Source: three-view drawing plus pictorial views. Frame: mm from the lowest corner of the part. A direction names the side the tool comes from. Give positions to 0.01 mm unless a question says otherwise; leave off trailing zeros. Write each loop counter-clockwise with the first axis right and the second up, starting at its lowest first coordinate (ties: lowest second). Pieces come first, ordered by that corner, then holes.
Q1. Reachability of the marked faces 5 and 6 from +Z, -Z, +X, -X, +Y, -Y: full face, straight path, thin tool, end or side. Return the list, or none.
Q2. Cut plane A-A on x = 11.75. Return the cut outline in (y, z).
Q3. Cut plane D-D on z = 1.3. Count the separate pieces of the cut face and the enclosed holes in it, plus the area to 3 significant figures.
Q4. Draft query along X for the marked faces 1, 2, 3 and 4. Return one class per face: pulls with the +X half, pulls with the -X half, needs draft (parallel to the pull), parting line crosses it, or undercut.
Q5. Line query: L1, parallel to X at y = 7.5, z = 0.5; L2, parallel to Y at x = 5.5, z = 1.75 (1 decimal); L3, parallel to Y at x = 5, z = 0.95 (1 decimal). Output: solid intervals per line, ascending.
Q6. Pin query (flat end, axial travel): pin 1 (0.7 mm diameter, centred on x = 10.5, z = 1.5, fed in from -Y); pin 2 (1 mm diameter, centred on y = 12, z = 1.5, fed in from -X); pin 3 (1.1 mm diameter, centred on y = 10.5, z = 0.5, fed in from -X) (1 decimal); pin 4 (0.5 mm diameter, centred on x = 7.5, z = 0.5, fed in from -Y). Return the tip coordinate at first contact, or that it passes through.
Q7. Cut plane C-C on x = 6. Return the cut outline in (y, z) (1 decimal).
Q8. Cut plane B-B on y = 13.25. Return the cut outline in (x, z).
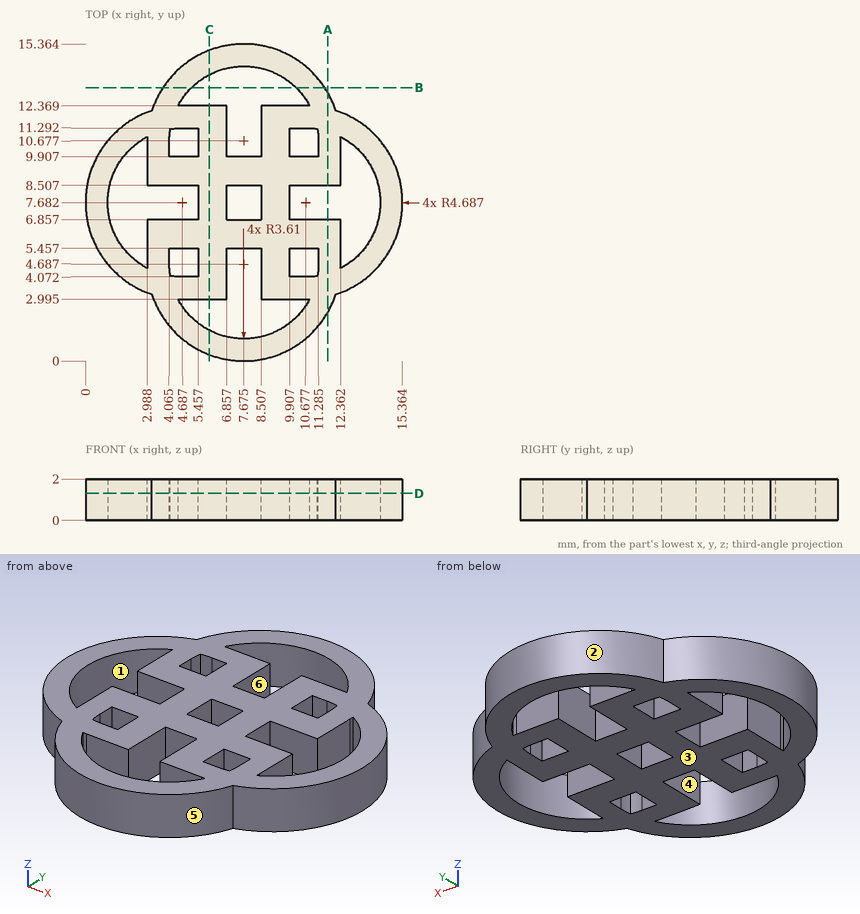
Data:
1. face 5: +Z, -Z, -Y
1. face 6: +Z, -Z
2. outline: (2.37, 0) - (6.86, 0) - (6.86, 2) - (2.37, 2) - close; (8.51, 0) - (12.99, 0) - (12.99, 2) - (8.51, 2) - close
3. separate pieces: 1
3. enclosed holes: 9
3. area: 102 mm2
4. face 1: undercut
4. face 2: parting line crosses it
4. face 3: needs draft
4. face 4: undercut
5. L1: x = 0 to 1.08, 5.46 to 6.86, 8.51 to 9.91, 14.28 to 15.36
5. L2: y = 0.5 to 1.8, 3 to 12.4, 13.6 to 14.8
5. L3: y = 0.8 to 2.3, 3 to 4.1, 5.5 to 6.9, 8.5 to 9.9, 11.3 to 12.4, 13.1 to 14.5
6. pin 1: stops at y = 0.71
6. pin 2: stops at x = 1.97
6. pin 3: stops at x = 0.6
6. pin 4: stops at y = 0
7. outline: (0.3, 0) - (1.5, 0) - (1.5, 2) - (0.3, 2) - close; (3, 0) - (12.4, 0) - (12.4, 2) - (3, 2) - close; (13.9, 0) - (15.1, 0) - (15.1, 2) - (13.9, 2) - close
8. outline: (3.76, 0) - (5.14, 0) - (5.14, 2) - (3.76, 2) - close; (10.21, 0) - (11.59, 0) - (11.59, 2) - (10.21, 2) - close
